Could you check a few things on this model? Use its own coordinates, in mm. Coordinates: 2 decimals unless noted, no trailing zeros. Order: outer loops, then holes, each group sorted by start corner. A loop starts at its lowest first (then second) coordinate and runs counter-clockwise, first axis right, second up. Notation, with made-up numbers: (46.25, 61) - (50.25, 61) arc R16 ccw to (50.25, 71) - close; hole circle Ø5 at (69.5, 9.25). An arc over 180 degrees is marked (long way). Answer as CSV lines item,"result". Start each with the question number.
1. For pin 1 (4.5 mm diameter, centred on x = -27, y = 9, fed in from +Z), with a flat end and sliding along its axis, tell me the tip position at first contact or that it passes through.
2. I want a section at A-A, the plane x = 26.5. List the corners of the cut face in (y, z) for me, and give its area (3 significant figures).
3. I want a section at D-D, the plane z = 0.35. List the corners of the cut face in (x, y) for me, and give its area (3 significant figures).
4. I need wall thicknesses on probe 1 along Y at (x, z) = (-27, 0.15); probe 2 along Y at (x, z) = (26.5, 0.3); probe 3 along Y at (x, z) = (-25.5, 0.1). Which ranges of each line are inside material? Lowest first, please.
5. I want a section at B-B, the plane y = 0. List the corners of the cut face in (x, z) for me, and give its area (3 significant figures).
6. I want a section at C-C, the plane x = -27. List the corners of the cut face in (y, z) for me.
7. Thinking about a two-plate mould opening in X: for faces 1 (the face through (-1, 0, 0)), 2 (the face through (-26.44, 6.46, 0.25)), which applies, released by +X, released by -X, zero draft, split by the parting line, or undercut?
from build123d import *

# Parameters (mm, degrees)
SKETCH1_W                    = 74
SKETCH1_H                    = 30
BASE_FLANGE1_DEPTH           = 0.5
F_5_2_5_2_DIAMETER_HOLE1_D   = 5.2
F_12_2_12_2_DIAMETER_HOLE1_D = 12.2


# Sheet-metal steps are written as plain solids
with BuildPart() as part:
    # Sketch1 → Base-Flange1 (new body)
    with BuildSketch(Plane.XY):
        Rectangle(SKETCH1_W, SKETCH1_H)
    extrude(amount=BASE_FLANGE1_DEPTH)

    # Ø5.2 (5.2) Diameter Hole1 (through all)
    with Locations(Plane.XY.offset(0.5)):
        with Locations((-27, 9)):
            f_5_2_5_2_diameter_hole1 = Hole(F_5_2_5_2_DIAMETER_HOLE1_D / 2)

    # Mirror1: Ø5.2 (5.2) Diameter Hole1 across plane
    add(f_5_2_5_2_diameter_hole1.mirror(Plane.ZX), mode=Mode.SUBTRACT)

    # Ø12.2 (12.2) Diameter Hole1 (through all)
    with Locations(Plane.XY.offset(0.5)):
        with Locations((26.5, 0)):
            Hole(F_12_2_12_2_DIAMETER_HOLE1_D / 2)


solid = part.part
Solved:
1,pin 1,"passes through"
2,outline,"(-15, 0) - (-6.1, 0) - (-6.1, 0.5) - (-15, 0.5) - close; (6.1, 0) - (15, 0) - (15, 0.5) - (6.1, 0.5) - close"
2,area,"8.90 mm2"
3,outline,"(-37, -15) - (37, -15) - (37, 15) - (-37, 15) - close; hole circle Ø5.2 at (-27, -9); hole circle Ø5.2 at (-27, 9); hole circle Ø12.2 at (26.5, 0)"
3,area,"2,060 mm2"
4,probe 1,"y = -15 to -11.6, -6.4 to 6.4, 11.6 to 15"
4,probe 2,"y = -15 to -6.1, 6.1 to 15"
4,probe 3,"y = -15 to -11.12, -6.88 to 6.88, 11.12 to 15"
5,outline,"(-37, 0) - (20.4, 0) - (20.4, 0.5) - (-37, 0.5) - close; (32.6, 0) - (37, 0) - (37, 0.5) - (32.6, 0.5) - close"
5,area,"30.9 mm2"
6,outline,"(-15, 0) - (-11.6, 0) - (-11.6, 0.5) - (-15, 0.5) - close; (-6.4, 0) - (6.4, 0) - (6.4, 0.5) - (-6.4, 0.5) - close; (11.6, 0) - (15, 0) - (15, 0.5) - (11.6, 0.5) - close"
7,face 1,"zero draft"
7,face 2,"undercut"
